Geometry check sheet. Reference: drawing and pictorial views, mm from the part's lowest x, y, z. A direction names the side the tool comes from. Give positions to 0.01 mm unless a question says otherwise; leave off trailing zeros. Write each loop counter-clockwise with the first axis right and the second up, starting at its lowest first coordinate (ties: lowest second). Pieces come first, ordered by that corner, then holes. Notation, with made-up numbers: M -2,10.5 L 49,10.5 A21 ccw 49,22.5 Z; hole C -11.75,89 d10. An arc over 180 degrees is marked long. Answer as a JSON object with one key per item and string values.
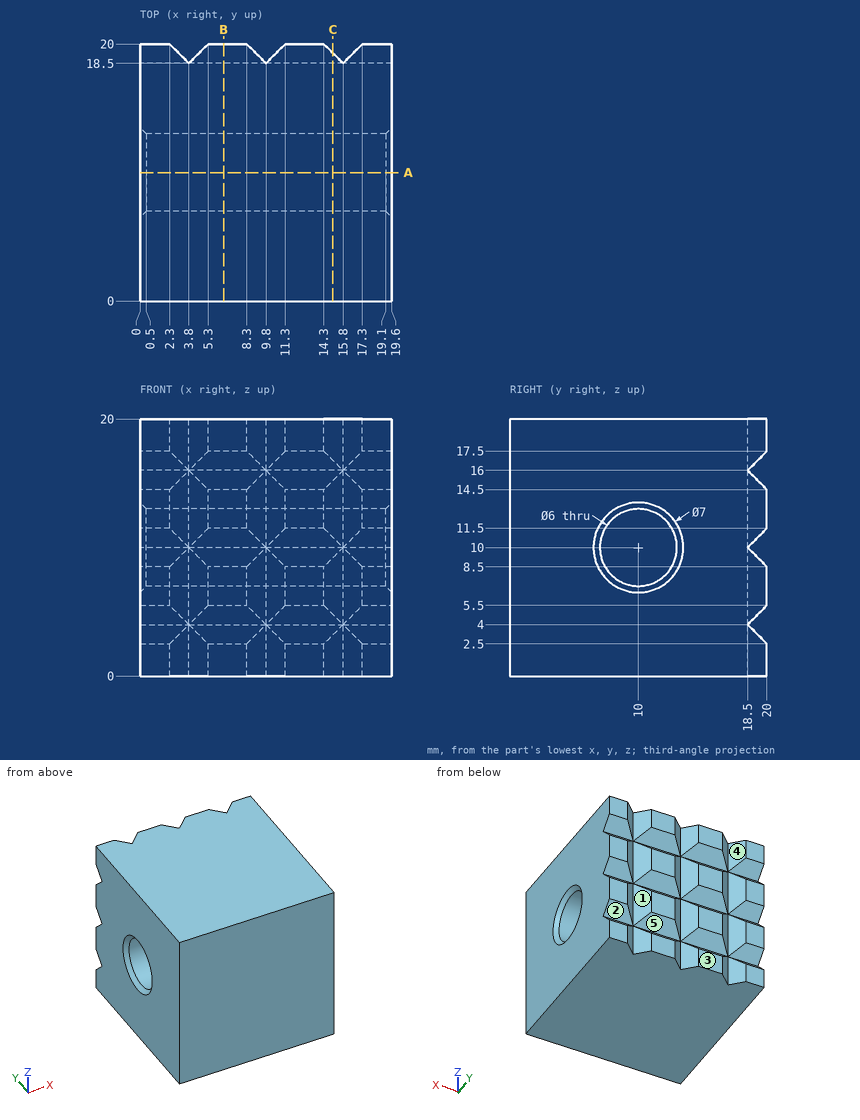
1) Section check A-A on y = 10. Record the boundary of the cut face in (x, z), and give its area (3 significant figures).
Completed:
{"outline": "M 0,0 L 19.6,0 L 19.6,6.5 L 19.1,7 L 0.5,7 L 0,6.5 Z; M 0,13.5 L 0.5,13 L 19.1,13 L 19.6,13.5 L 19.6,20 L 0,20 Z", "area": "274 mm2"}
2) Section check C-C on x = 15. Record the boundary of the cut face in (y, z).
Completed:
{"outline": "M 0,0 L 19.3,0 L 19.3,3.2 L 18.5,4 L 19.3,4.8 L 19.3,9.2 L 18.5,10 L 19.3,10.8 L 19.3,15.2 L 18.5,16 L 19.3,16.8 L 19.3,20 L 0,20 Z; hole C 10,10 d6"}
3) Release check for a two-part mould opening along X. For the marked faces 4 and 5 record: pulls with the +X half, pulls with the -X half, needs draft (parallel to the pull), parting line crosses it, or undercut.
Completed:
{"face 4": "undercut", "face 5": "needs draft"}
4) Section check B-B on x = 6.5. Record the boundary of the cut face in (y, z), and give its area (3 significant figures).
Completed:
{"outline": "M 0,0 L 20,0 L 20,2.5 L 18.5,4 L 20,5.5 L 20,8.5 L 18.5,10 L 20,11.5 L 20,14.5 L 18.5,16 L 20,17.5 L 20,20 L 0,20 Z; hole C 10,10 d6", "area": "365 mm2"}
5) Thickness scan on L1, parallel to Y at x = 17.5, z = 9; L2, parallel to Z at x = 5, y = 9.75; L3, parallel to Z at x = 19.25, y = 10.75. Record the ranges inside material, lowest first.
Completed:
{"L1": "y = 0 to 7.17, 12.83 to 19.5", "L2": "z = 0 to 7.01, 12.99 to 20", "L3": "z = 0 to 6.94, 13.06 to 20"}
6) Access from +Z, -Z, +X, -X, +Y, -Y to the whole of each face (thin tool, end or side, straight path). Record for the marked faces 1, 2 and 3.
Completed:
{"face 1": "+Z, -Z, +Y", "face 2": "+X, -X, +Y", "face 3": "+Z, -Z, +X, -X, +Y"}
